from build123d import *

# Parameters (mm, degrees)
SKETCH1_W           = 80
SKETCH1_H           = 160
BOSS_EXTRUDE1_DEPTH = 25
SKETCH2_R           = 100
CUT_EXTRUDE1_DEPTH  = 181.623918682
FILLET1_R           = 10
SHELL1_T            = -2
SKETCH3_R           = 4
BOSS_EXTRUDE2_DEPTH = 23
SKETCH6_R           = 2
CUT_EXTRUDE2_DEPTH  = 10
SKETCH7_R           = 3
BOSS_EXTRUDE3_DEPTH = 23
SKETCH8_W           = 15
SKETCH8_H           = 9
CUT_EXTRUDE3_DEPTH  = 10


with BuildPart() as part:
    # Sketch1 → Boss-Extrude1 (new body)
    with BuildSketch(Plane(origin=(0, 0, 0), x_dir=(1, 0, 0), z_dir=(0, 1, 0))):
        with Locations((40, 80)):
            Rectangle(SKETCH1_W, SKETCH1_H)
    extrude(amount=-BOSS_EXTRUDE1_DEPTH)

    # Sketch2 → Cut-Extrude1 (cut, through all)
    with BuildSketch(Plane(origin=(0, 0, 0), x_dir=(1, 0, 0), z_dir=(0, 1, 0))):
        with Locations((-95, 80)):
            Circle(SKETCH2_R)
        with Locations((175, 80)):
            Circle(SKETCH2_R)
    extrude(amount=-CUT_EXTRUDE1_DEPTH, mode=Mode.SUBTRACT)

    # Fillet1
    fillet1_edges = [part.edges().sort_by_distance(p)[0] for p in [
        (0, -12.5, -160),
        (80, -12.5, -160),
        (80, -12.5, 0),
        (0, -12.5, 0),
    ]]
    fillet(fillet1_edges, radius=FILLET1_R)

    # Shell1
    shell1_openings = [part.faces().sort_by_distance(p)[0] for p in [
        (40, 0, -80),
    ]]
    offset(amount=SHELL1_T, openings=shell1_openings, kind=Kind.INTERSECTION)

    # Sketch3 → Boss-Extrude2 (add, through all)
    with BuildSketch(Plane(origin=(0, -23, 0), x_dir=(1, 0, 0), z_dir=(0, 1, 0))):
        with Locations(Location((10, 150, 0), (0, 0, 90))):
            Circle(SKETCH3_R)
        with Locations(Location((70, 150, 0), (0, 0, 90))):
            Circle(SKETCH3_R)
        with Locations(Location((70, 10, 0), (0, 0, 90))):
            Circle(SKETCH3_R)
        with Locations(Location((10, 10, 0), (0, 0, 90))):
            Circle(SKETCH3_R)
    extrude(amount=BOSS_EXTRUDE2_DEPTH)

    # Sketch6 → Cut-Extrude2 (cut)
    with BuildSketch(Plane(origin=(0, 0, 0), x_dir=(1, 0, 0), z_dir=(0, 1, 0))):
        with Locations(Location((10, 150, 0), (0, 0, 270))):
            Circle(SKETCH6_R)
        with Locations(Location((70, 150, 0), (0, 0, 90))):
            Circle(SKETCH6_R)
        with Locations(Location((70, 10, 0), (0, 0, 270))):
            Circle(SKETCH6_R)
        with Locations(Location((10, 10, 0), (0, 0, 90))):
            Circle(SKETCH6_R)
    extrude(amount=-CUT_EXTRUDE2_DEPTH, mode=Mode.SUBTRACT)

    # Sketch7 → Boss-Extrude3 (add, through all)
    with BuildSketch(Plane(origin=(0, -23, 0), x_dir=(1, 0, 0), z_dir=(0, 1, 0))):
        with Locations(Location((14, 121, 0), (0, 0, 90))):
            Circle(SKETCH7_R)
        with Locations(Location((66, 121, 0), (0, 0, 90))):
            Circle(SKETCH7_R)
        with Locations(Location((14, 19, 0), (0, 0, 90))):
            Circle(SKETCH7_R)
        with Locations(Location((66, 19, 0), (0, 0, 90))):
            Circle(SKETCH7_R)
    extrude(amount=BOSS_EXTRUDE3_DEPTH)

    # Sketch8 → Cut-Extrude3 (cut)
    with BuildSketch(Plane(origin=(80, 0, 0), x_dir=(0, 0, -1), z_dir=(1, 0, 0))):
        with Locations((134.724989992, -12.5)):
            Rectangle(SKETCH8_W, SKETCH8_H)
    extrude(amount=-CUT_EXTRUDE3_DEPTH, mode=Mode.SUBTRACT)


solid = part.part
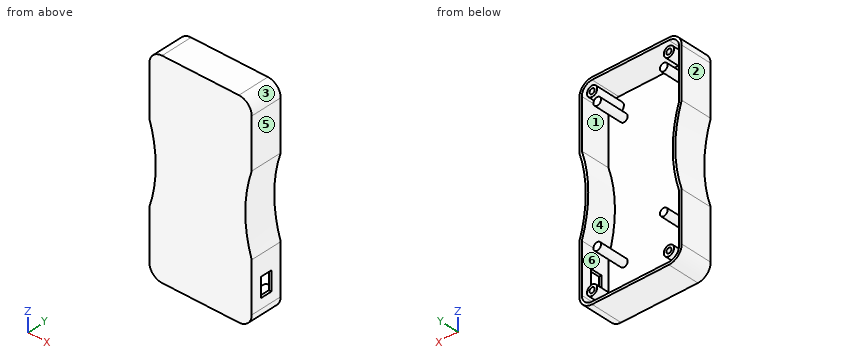
Here's how the part is built. I have some questions about the finished solid (model axes, mm). Face numbers are marked on the shaded views. A direction names the side the tool comes from. Coordinates: 2 decimals unless noted, no trailing zeros. Write each loop counter-clockwise with the first axis right and the second up, starting at its lowest first coordinate (ties: lowest second). Pieces come first, ordered by that corner, then holes.
1) Which directions (+Z, -Z, +X, -X, +Y, -Y) give clear straight access to the entire face, cutting with the end or side of a thin tool? Please do the marked faces 1 and 2.
Filled in:
face 1: +Y
face 2: +Z, -Z, -X, +Y, -Y
2) If I drill on line 1 (X direction, y = -6.5, z = -150); line 2 (Z direction, x = 34, y = -13.25); line 3 (X direction, y = -18, z = -132.5), over which ranges is the centre line in solid material (lowest first)?
Filled in:
line 1: x = 0 to 2, 6 to 8, 12 to 14, 66 to 68, 72 to 74, 78 to 80
line 2: z = -160 to -158, -2 to 0
line 3: x = 0 to 2, 78 to 80
3) If we section it at C-C (x = 23): List the corners of the cut face in (y, z) for me.
Filled in:
outline: (-25, -160) - (0, -160) - (0, -158) - (-23, -158) - (-23, -2) - (0, -2) - (0, 0) - (-25, 0) - close
4) If we section it at B-B (z = -30): List the corners of the cut face in (x, y) for me.
Filled in:
outline: (0, -25) - (80, -25) - (80, 0) - (78, 0) - (78, -23) - (2, -23) - (2, 0) - (0, 0) - close
5) I'm going to push flat-ended pins straight in: pin 1 (1 mm diameter, centred on x = 79.5, y = -11, fed in from -Z); pin 2 (3 mm diameter, centred on x = 10, z = -150, fed in from +Y); pin 3 (1.5 mm diameter, centred on x = 70, z = -141, fed in from +Y). Where does each tip first touch, or does it pass through?
Filled in:
pin 1: stops at z = -154.36
pin 2: stops at y = -10
pin 3: stops at y = -23
6) Thinking about a two-plate mould opening in Z: for the marked faces 3, 4, 5 and 6, which applies, +Z half, -Z half, draft (parallel to the pull), parting line (faces both ways), or undercut?
Filled in:
face 3: +Z half
face 4: undercut
face 5: draft
face 6: undercut
7) If we section it at A-A (y = -18.5): Count the separate pieces of the cut face and the enclosed holes in it, plus the area to 3 significant figures.
Filled in:
separate pieces: 9
enclosed holes: 1
area: 1,230 mm2
